Geometry: see drawing. Coordinates: mm, zero at the bounding-box minimum. A direction names the side the tool comes from. Give positions to 0.01 mm unless a question says otherwise; leave off trailing zeros. Write each loop counter-clockwise with the first axis right and the second up, starting at its lowest first coordinate (ties: lowest second). Pieces come first, ordered by that corner, then holes. Notation, with made-up numbers: (40.5, 42) - (44.5, 42) arc R20 ccw to (44.5, 61) - close; hole circle Ø10 at (75, -5.75). An arc over 180 degrees is marked (long way). Use a Markdown table: item, result. Add a question column.
1. Set-up query: the marked faces 1, 2 and 3. Return all of +Z, -Z, +X, -X, +Y, -Y with unobstructed straight access to the full face (end or side cutting, diameter ignored); none if empty.
2. Section query C-C, the plane y = 15. Return loops of the section in (x, z), plus the area to 3 significant figures.
3. Mould query, pull axis X, two halves, no side actions, for the marked faces 4, 5 and 6. Classes: released by +X, released by -X, zero draft, split by the parting line, or undercut.
4. Section query B-B, the plane z = 1.1. Return loops of the section in (x, y).
5. Material intervals for probe 1 along X at (y, z) = (15, 0.6); probe 2 along Y at (x, z) = (4, 3.5); probe 3 along Y at (x, z) = (4, 0.65), sorted ascending.
6. Section query D-D, the plane z = 3. Return loops of the section in (x, y).
7. Section query A-A, the plane x = 4. Return loops of the section in (y, z).
8. Pin query (flat end, axial travel): pin 1 (2.5 mm diameter, centred on x = 12, y = 15, fed in from +Z); pin 2 (1 mm diameter, centred on x = 4, z = 1.5, fed in from -Y). Return the tip coordinate at first contact, or that it passes through.
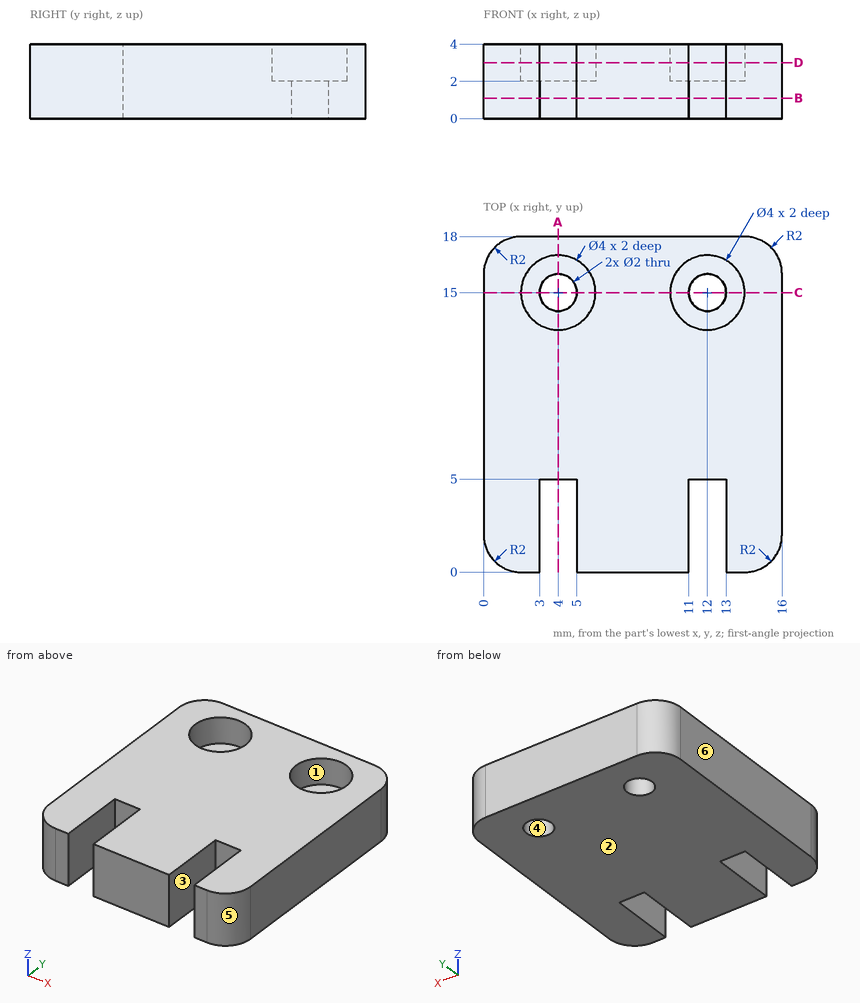
Result sheet:
| question | item | result |
|---|---|---|
| 1 | face 1 | +Z |
| 1 | face 2 | -Z, +X, -X, +Y, -Y |
| 1 | face 3 | +Z, -Z, -Y |
| 2 | outline | (0, 0) - (3, 0) - (3, 2) - (2, 2) - (2, 4) - (0, 4) - close; (5, 0) - (11, 0) - (11, 2) - (10, 2) - (10, 4) - (6, 4) - (6, 2) - (5, 2) - close; (13, 0) - (16, 0) - (16, 4) - (14, 4) - (14, 2) - (13, 2) - close |
| 2 | area | 40.0 mm² |
| 3 | face 4 | undercut |
| 3 | face 5 | released by +X |
| 3 | face 6 | released by -X |
| 4 | outline | (0, 2) arc R2 ccw to (2, 0) - (3, 0) - (3, 5) - (5, 5) - (5, 0) - (11, 0) - (11, 5) - (13, 5) - (13, 0) - (14, 0) arc R2 ccw to (16, 2) - (16, 16) arc R2 ccw to (14, 18) - (2, 18) arc R2 ccw to (0, 16) - close; hole circle Ø2 at (4, 15); hole circle Ø2 at (12, 15) |
| 5 | probe 1 | x = 0 to 3, 5 to 11, 13 to 16 |
| 5 | probe 2 | y = 5 to 13, 17 to 18 |
| 5 | probe 3 | y = 5 to 14, 16 to 18 |
| 6 | outline | (0, 2) arc R2 ccw to (2, 0) - (3, 0) - (3, 5) - (5, 5) - (5, 0) - (11, 0) - (11, 5) - (13, 5) - (13, 0) - (14, 0) arc R2 ccw to (16, 2) - (16, 16) arc R2 ccw to (14, 18) - (2, 18) arc R2 ccw to (0, 16) - close; hole circle Ø4 at (4, 15); hole circle Ø4 at (12, 15) |
| 7 | outline | (5, 0) - (14, 0) - (14, 2) - (13, 2) - (13, 4) - (5, 4) - close; (16, 0) - (18, 0) - (18, 4) - (17, 4) - (17, 2) - (16, 2) - close |
| 8 | pin 1 | stops at z = 2 |
| 8 | pin 2 | stops at y = 5 |
